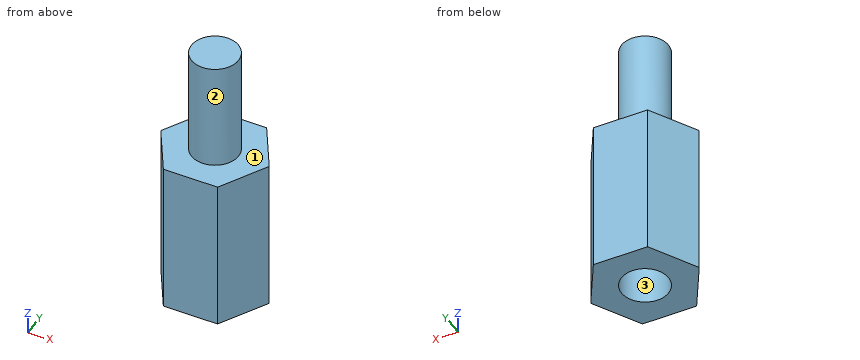
```python
from build123d import *

# Parameters (mm, degrees)
F1_DEPTH = 10
F2_R     = 1.5
F3_DEPTH = 7
F4_R     = 1.5
F5_DEPTH = 5


with BuildPart() as f1:
    # F0 (on Top) → F1 (new body)
    with BuildSketch(Plane.XY):
        Polygon((1.7320508076, 3), (-1.7320508076, 3), (-3.4641016151, 0), (-1.7320508076, -3), (1.7320508076, -3), (3.4641016151, 0), align=None)
    extrude(amount=F1_DEPTH)

    # F2 (on face) → F3 (join)
    with BuildSketch(Plane.XY.offset(10)):
        Circle(F2_R)
    extrude(amount=F3_DEPTH)

    # F4 (on face) → F5 (cut)
    with BuildSketch(Plane(origin=(0, 0, 0), x_dir=(1, 0, 0), z_dir=(0, 0, -1))):
        Circle(F4_R)
    extrude(amount=-F5_DEPTH, mode=Mode.SUBTRACT)


solid = f1.part
```
The model under review builds one solid part; all positions refer to its coordinate system, in mm. Face numbers are marked on the shaded views. Give positions to 0.01 mm unless a question says otherwise; leave off trailing zeros. Write each loop counter-clockwise with the first axis right and the second up, starting at its lowest first coordinate (ties: lowest second). Pieces come first, ordered by that corner, then holes. Notation, with made-up numbers: (15, 53) -> (27, 53) arc R16 ccw to (27, 80) -> close; hole circle Ø5 at (89, 35). An arc over 180 degrees is marked (long way). Put each result on its own line as item: value.
(1) We need section B-B, the plane x = 0. Give the boundary of the cut face in (y, z).
Results are:
outline: (-3, 0) -> (-1.5, 0) -> (-1.5, 5) -> (1.5, 5) -> (1.5, 0) -> (3, 0) -> (3, 10) -> (1.5, 10) -> (1.5, 17) -> (-1.5, 17) -> (-1.5, 10) -> (-3, 10) -> close
(2) For pin 1 Ø1.5 at (x, y) = (0, 0.5) entering from -Z; pin 2 Ø1.5 at (y, z) = (1, 4) entering from -X, all flat-tipped, find the tip position at first contact; note any pin that passes through.
Results are:
pin 1: z = 5
pin 2: x = -3.32
(3) We need section C-C, the plane y = 1. Give the boundary of the cut face in (x, z), and give its area (3 significant figures).
Results are:
outline: (-2.89, 0) -> (-1.12, 0) -> (-1.12, 5) -> (1.12, 5) -> (1.12, 0) -> (2.89, 0) -> (2.89, 10) -> (1.12, 10) -> (1.12, 17) -> (-1.12, 17) -> (-1.12, 10) -> (-2.89, 10) -> close
area: 62.2 mm²
(4) We need section A-A, the plane z = 1.5. Give the boundary of the cut face in (x, y).
Results are:
outline: (-3.46, 0) -> (-1.73, -3) -> (1.73, -3) -> (3.46, 0) -> (1.73, 3) -> (-1.73, 3) -> close; hole circle Ø3 at (0, 0)
(5) The part is to be moulded in two halves that separate along X. For the marked faces 1, 2 and 3, say which applies: pulls with the +X half, pulls with the -X half, needs draft (parallel to the pull), parting line crosses it, or undercut.
Results are:
face 1: needs draft
face 2: parting line crosses it
face 3: undercut
(6) To check wall thickness, follow probe 1 along Y at (x, z) = (0, 1.9); probe 2 along Z at (x, y) = (1.5, -1); probe 3 along X at (y, z) = (1, 2.25). State the ranges of each line that lie inside material, in increasing order. Write a range as from..to.
Results are:
probe 1: -3..-1.5, 1.5..3
probe 2: 0..10
probe 3: -2.89..-1.12, 1.12..2.89
(7) We need section D-D, the plane z = 9.75. Give the boundary of the cut face in (x, y).
Results are:
outline: (-3.46, 0) -> (-1.73, -3) -> (1.73, -3) -> (3.46, 0) -> (1.73, 3) -> (-1.73, 3) -> close
